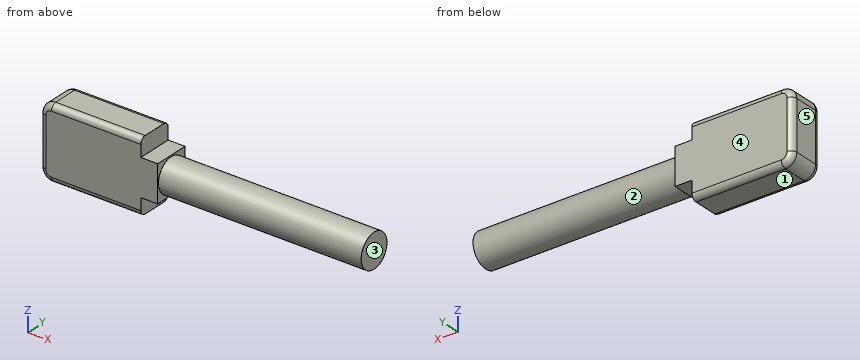
```python
from build123d import *

# Parameters (mm, degrees)
PAD002_DEPTH = 3.175
FILLET001_R  = 2
FILLET002_R  = 1
SKETCH010_R  = 3
PAD003_DEPTH = 36


with BuildPart() as part:
    # Sketch009 → Pad002 (new body, symmetric)
    with BuildSketch(Plane.XZ):
        Polygon((0, 3.25), (-3, 3.25), (-3, 6.35), (-20.8816, 6.35), (-20.8816, 0), (0, 0), align=None)
    pad002 = extrude(amount=PAD002_DEPTH, both=True)

    # Mirrored: Pad002 across Sketch009 H_Axis
    add(pad002.mirror(Plane(origin=(0, 0, 0), x_dir=(0, -1, 0), z_dir=(0, 0, 1))))

    # Fillet001
    fillet001_edges = [part.edges().sort_by_distance(p)[0] for p in [
        (-20.8816, 0, -6.35),
        (-20.8816, 0, 6.35),
    ]]
    fillet(fillet001_edges, radius=FILLET001_R)

    # Fillet002
    fillet002_edges = [part.edges().sort_by_distance(p)[0] for p in [
        (-10.9408, 3.175, 6.35),
        (-10.9408, -3.175, 6.35),
    ]]
    fillet(fillet002_edges, radius=FILLET002_R)

    # Sketch010 → Pad003 (join)
    with BuildSketch(Plane.YZ):
        Circle(SKETCH010_R)
    extrude(amount=PAD003_DEPTH)


solid = part.part
```
Read the model definition and answer for the solid it produces. Units are mm, in the model's axes. Face numbers are marked on the shaded views. A direction names the side the tool comes from. Give positions to 0.01 mm unless a question says otherwise; leave off trailing zeros. Order: outer loops, then holes, each group sorted by start corner. A loop starts at its lowest first (then second) coordinate and runs counter-clockwise, first axis right, second up.
(1) Find section C-C (x = 18). Give the vertices of the cut face in (y, z).
(2) Find section B-B (y = 0). Give the vertices of the cut face in (x, z).
(3) For a pull along X with two mould halves and no side action, classify the marked faces 3, 4 and 5 as released by +X, released by -X, zero draft, split by the parting line, or undercut.
(4) Find section A-A (z = 0). Give the vertices of the cut face in (x, y) (3 decimals).
(5) Straight lines are drawn through the part: L1, parallel to Z at x = -5, y = 2.25; L2, parallel to X at y = 0, z = 3.5; L3, parallel to Z at x = -2.5, y = 0.25. For each, find the intervals that lie inside material, in ascending order.
(6) For the marked faces 1 and 2, determine the directions among +Z, -Z, +X, -X, +Y, -Y from which every point of the face is accessible in a straight line to the end or side of a thin tool.
(7) Given pin 1 (2 mm diameter, centred on x = 19.5, y = 1.5, fed in from +Z); pin 2 (6 mm diameter, centred on x = 8, z = -2, fed in from -Y); pin 3 (1.5 mm diameter, centred on x = 23.5, y = 1, fed in from -Z), each flat-ended and moving along its own axis, determine where each tip first touches the part or whether it passes through.
Result sheet:
1. outline: circle Ø6 at (0, 0)
2. outline: (-20.88, -4.35) arc R2 ccw to (-18.88, -6.35) - (-3, -6.35) - (-3, -3.25) - (0, -3.25) - (0, -3) - (36, -3) - (36, 3) - (0, 3) - (0, 3.25) - (-3, 3.25) - (-3, 6.35) - (-18.88, 6.35) arc R2 ccw to (-20.88, 4.35) - close
3. face 3: released by +X
3. face 4: zero draft
3. face 5: released by -X
4. outline: (-20.882, -2.175) arc R1 ccw to (-19.882, -3.175) - (0, -3.175) - (0, -3) - (36, -3) - (36, 3) - (0, 3) - (0, 3.175) - (-19.882, 3.175) arc R1 ccw to (-20.882, 2.175) - close
5. L1: z = -6.35 to 6.35
5. L2: x = -20.88 to -3
5. L3: z = -3.25 to 3.25
6. face 1: -Z, +X, -X, +Y, -Y
6. face 2: +X
7. pin 1: stops at z = 2.96
7. pin 2: stops at y = -3
7. pin 3: stops at z = -2.99
